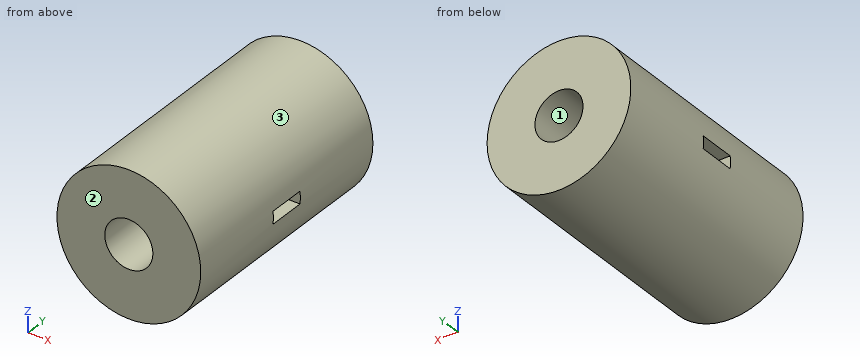
from build123d import *

# Parameters (mm, degrees)
F0_R     = 45
F1_DEPTH = 75
F2_R     = 15.05
F3_DEPTH = 150
F4_W     = 23.5
F4_H     = 7.8
F5_DEPTH = 63


with BuildPart() as f1:
    # F0 (on Front) → F1 (new body, symmetric)
    with BuildSketch(Plane.XZ):
        Circle(F0_R)
    extrude(amount=F1_DEPTH, both=True)

    # F2 (on face) → F3 (cut, symmetric)
    with BuildSketch(Plane.XZ.offset(75)):
        Circle(F2_R)
    extrude(amount=F3_DEPTH, both=True, mode=Mode.SUBTRACT)

    # F4 (on Right) → F5 (cut, symmetric)
    with BuildSketch(Plane.YZ):
        Rectangle(F4_W, F4_H)
    extrude(amount=F5_DEPTH, both=True, mode=Mode.SUBTRACT)


solid = f1.part
Geometry: final body of the model. Coordinates: model frame, mm. Face numbers are marked on the shaded views. Round coordinates to 2 decimals unless told otherwise and drop trailing zeros. Loops run counter-clockwise (first coordinate to the right, second up) from the corner with the lowest first, then second, coordinate; pieces in that order, holes last. Notation, with made-up numbers: (29, 60) - (36, 60) arc R11 ccw to (36, 80) - close; hole circle Ø11 at (-12.5, 67.5). An arc over 180 degrees is marked (long way). Write each question's results on one line, items separated by ' | '. Start each with the question number.
1) Cut plane B-B on z = 0. Return loops of the section in (x, y).
2) Cut plane C-C on y = -46. Return loops of the section in (x, z).
3) Mould query, pull axis Z, two halves, no side actions, for the marked faces 1, 2 and 3. Classes: released by +Z, released by -Z, zero draft, split by the parting line, or undercut.
4) Cut plane D-D on x = -20. Return loops of the section in (y, z).
5) First-contact query: P1, Ø7, axis at x = 27.5, y = 1, coming from the +Z side; P2, Ø8, axis at y = 34.5, z = 25, coming from the +X side; P3, Ø18, axis at x = 0, z = 0, coming from the +Y side; P4, Ø6, axis at x = 19, y = -14.5, coming from the -Z side. Flat tips, straight axial feed; report the tip coordinate or a pass-through.
6) Line query: probe 1 along Y at (x, z) = (-35.5, 2.5); probe 2 along Z at (x, y) = (0, 6); probe 3 along X at (y, z) = (-38, 3.5). Output: solid intervals per line, ascending. Write a range as [from, to].
7) Cut plane A-A on x = 0. Return loops of the section in (y, z), then the cut area to 4 significant figures.
Verdict:
1) outline: (-45, -75) - (-15.05, -75) - (-15.05, -11.75) - (-45, -11.75) - close; (-45, 11.75) - (-15.05, 11.75) - (-15.05, 75) - (-45, 75) - close; (15.05, -75) - (45, -75) - (45, -11.75) - (15.05, -11.75) - close; (15.05, 11.75) - (45, 11.75) - (45, 75) - (15.05, 75) - close
2) outline: circle Ø90 at (0, 0); hole circle Ø30.1 at (0, 0)
3) face 1: undercut | face 2: zero draft | face 3: split by the parting line
4) outline: (-75, -40.31) - (75, -40.31) - (75, 40.31) - (-75, 40.31) - close; hole (-11.75, -3.9) - (11.75, -3.9) - (11.75, 3.9) - (-11.75, 3.9) - close
5) P1: stops at z = 38.07 | P2: stops at x = 39.8 | P3: passes through | P4: stops at z = -42.06
6) probe 1: y = [-75, -11.75], [11.75, 75] | probe 2: z = [-45, -15.05], [15.05, 45] | probe 3: x = [-44.86, -14.64], [14.64, 44.86]
7) outline: (-75, -45) - (75, -45) - (75, -15.05) - (-75, -15.05) - close; (-75, 15.05) - (75, 15.05) - (75, 45) - (-75, 45) - close | area: 8,985 mm2
